```python
from build123d import *

# Parameters (mm, degrees)
BOSS_EXTRUDE1_DEPTH              = 19.05
CUT_EXTRUDE2_DEPTH               = 7658.473916494
FILLET1_R                        = 76.2
FILLET2_R                        = 31.75
SKETCH2_W                        = 127
SKETCH2_H                        = 19.05
CUT_EXTRUDE1_DEPTH               = 7658.473916494
F_1_4_0_25_DIAMETER_HOLE1_D      = 6.35
F_15_64_0_23438_DIAMETER_HOLE1_D = 5.953252
F_1_4_CLEARANCE_HOLE1_D          = 7.14248
HOLE1_D                          = 3.175
HOLE1_DEPTH                      = 50.8
HOLE1_CSINK_D                    = 10.16
HOLE1_CSINK_ANGLE                = 82
HOLE1_TIP                        = 0.953866233
HOLE2_D                          = 3.175
HOLE2_DEPTH                      = 38.1
HOLE2_CSINK_D                    = 10.16
HOLE2_CSINK_ANGLE                = 82
HOLE2_TIP                        = 0.953866233
HOLE3_D                          = 3.175
HOLE3_DEPTH                      = 50.8
HOLE3_CSINK_D                    = 10.16
HOLE3_CSINK_ANGLE                = 82
HOLE3_TIP                        = 0.953866233
HOLE4_D                          = 3.175
HOLE4_DEPTH                      = 38.1
HOLE4_CSINK_D                    = 10.16
HOLE4_CSINK_ANGLE                = 82
HOLE4_TIP                        = 0.953866233


with BuildPart() as part:
    # Sketch1 → Boss-Extrude1 (new body)
    with BuildSketch(Plane.XY):
        Polygon((3140.71, 6983.72999014), (2683.51, 6983.72999014), (2683.51, 6641.741886848), (3140.71, 6826.4626773), align=None)
    extrude(amount=BOSS_EXTRUDE1_DEPTH)

    # Sketch6 → Cut-Extrude2 (cut, through all)
    with BuildSketch(Plane(origin=(0, 0, 0), x_dir=(-1, 0, 0), z_dir=(0, 0, -1))):
        Polygon((-2923.76447292, 6932.92999014), (-3089.91, 6932.92999014), (-3089.91, 6860.727709955), (-2972.15765047, 6813.152672592), align=None)
        Polygon((-2925.056710658, 6794.122657646), (-2734.31, 6717.055984048), (-2734.31, 6932.92999014), (-2868.974907992, 6932.92999014), align=None)
    extrude(amount=-CUT_EXTRUDE2_DEPTH, mode=Mode.SUBTRACT)

    # Fillet1
    fillet1_edges = [part.edges().sort_by_distance(p)[0] for p in [
        (2925.056710658, 6794.122657646, 9.525),
        (2868.974907992, 6932.92999014, 9.525),
        (2734.31, 6932.92999014, 9.525),
        (2734.31, 6717.055984048, 9.525),
    ]]
    fillet(fillet1_edges, radius=FILLET1_R)

    # Fillet2
    fillet2_edges = [part.edges().sort_by_distance(p)[0] for p in [
        (2972.15765047, 6813.152672592, 9.525),
        (3089.91, 6860.727709955, 9.525),
        (3089.91, 6932.92999014, 9.525),
        (2923.76447292, 6932.92999014, 9.525),
    ]]
    fillet(fillet2_edges, radius=FILLET2_R)

    # Sketch2 → Cut-Extrude1 (cut, through all)
    with BuildSketch(Plane(origin=(0, 0, 0), x_dir=(-1, 0, 0), z_dir=(0, 0, -1))):
        with Locations((-2747.01, 6974.20499014)):
            Rectangle(SKETCH2_W, SKETCH2_H)
        with Locations((-3001.01, 6974.20499014)):
            Rectangle(SKETCH2_W, SKETCH2_H)
        Polygon((-2977.551881268, 6760.542518374), (-3095.304230798, 6808.117555738), (-3088.167975193, 6825.780408168), (-2970.415625663, 6778.205370804), align=None)
    extrude(amount=-CUT_EXTRUDE1_DEPTH, mode=Mode.SUBTRACT)

    # 1/4 (0.25) Diameter Hole1 (through all)
    with Locations(Plane(origin=(0, 0, 0), x_dir=(-1, 0, 0), z_dir=(0, 0, -1))):
        with Locations((-3088.167975193, 6825.780408168), (-2970.415625663, 6778.205370804), (-2937.51, 6964.67999014), (-3064.51, 6964.67999014), (-2810.51, 6964.67999014)):
            Hole(F_1_4_0_25_DIAMETER_HOLE1_D / 2)

    # 15/64 (0.23438) Diameter Hole1 (through all)
    with Locations(Plane.YX):
        with Locations((6692.541891629, 2721.610000001), (6945.629994921, 2721.610000001), (6945.629994921, 3115.310000001), (6851.60701674, 3115.310000001)):
            Hole(F_15_64_0_23438_DIAMETER_HOLE1_D / 2)

    # 1/4 Clearance Hole1 (through all)
    with Locations(Plane(origin=(0, 0, 0), x_dir=(-1, 0, 0), z_dir=(0, 0, -1))):
        with Locations((-2900.218040257, 6923.40499014)):
            Hole(F_1_4_CLEARANCE_HOLE1_D / 2)

    # Hole1
    with Locations(Plane(origin=(0, 7002.77999014, 247.523), x_dir=(0, 0, 1), z_dir=(0, 1, 0))):
        with Locations((0, 2696.21), (-237.998, 3089.91), (-237.998, 3039.11), (-237.998, 2962.91), (-237.998, 2912.11), (-237.998, 2835.91), (-237.998, 2785.11), (-237.998, 2708.91), (237.998, 2708.91), (237.998, 2785.11), (237.998, 2835.91), (237.998, 2912.11), (237.998, 2962.91), (237.998, 3039.11), (237.998, 3089.91), (0, 3051.81), (0, 2950.21), (0, 2797.81)):
            CounterSinkHole(HOLE1_D / 2, HOLE1_CSINK_D / 2, depth=HOLE1_DEPTH, counter_sink_angle=HOLE1_CSINK_ANGLE)
            with Locations((0, 0, -(HOLE1_DEPTH + HOLE1_TIP / 2))):  # 118° drill point
                Cone(0, HOLE1_D / 2, HOLE1_TIP, mode=Mode.SUBTRACT)

    # Hole2
    with Locations(Plane(origin=(3159.76, -4.781e-06, 247.523), x_dir=(0, 0, -1), z_dir=(1, 0, 0))):
        with Locations((-118.999, 6993.254994921), (237.998, 6993.254994921), (237.998, 6958.329994921), (237.998, 6845.512682081), (-237.998, 6993.254994921), (-237.998, 6958.329994921), (-237.998, 6845.512682081), (118.999, 6993.254994921)):
            CounterSinkHole(HOLE2_D / 2, HOLE2_CSINK_D / 2, depth=HOLE2_DEPTH, counter_sink_angle=HOLE2_CSINK_ANGLE)
            with Locations((0, 0, -(HOLE2_DEPTH + HOLE2_TIP / 2))):  # 118° drill point
                Cone(0, HOLE2_D / 2, HOLE2_TIP, mode=Mode.SUBTRACT)

    # Hole3
    with Locations(Plane(origin=(-1923.157317923, 4759.981389861, 247.523), x_dir=(0, 0, -1), z_dir=(0.37460659341595665, -0.9271838545667693, 0))):
        with Locations((237.998, 5442.50683469), (-237.998, 5442.50683469), (-237.998, 5394.88183469), (-237.998, 5318.68183469), (0, 5407.58183469), (0, 5305.98183469), (-237.998, 5267.88183469), (-237.998, 5130.866292514), (-237.998, 4993.850750338), (237.998, 4993.850750338), (237.998, 5130.866292514), (237.998, 5267.88183469), (237.998, 5318.68183469), (237.998, 5394.88183469)):
            CounterSinkHole(HOLE3_D / 2, HOLE3_CSINK_D / 2, depth=HOLE3_DEPTH, counter_sink_angle=HOLE3_CSINK_ANGLE)
            with Locations((0, 0, -(HOLE3_DEPTH + HOLE3_TIP / 2))):  # 118° drill point
                Cone(0, HOLE3_D / 2, HOLE3_TIP, mode=Mode.SUBTRACT)

    # Hole4
    with Locations(Plane(origin=(2664.46, -4.781e-06, 247.523), x_dir=(0, 0, 1), z_dir=(-1, 0, 0))):
        with Locations((-237.998, 6686.191891629), (237.998, 6686.191891629), (257.048, 6993.254994921), (218.948, 6993.254994921), (19.05, 6993.254994921), (237.998, 6939.279994921), (237.998, 6812.735943275), (-237.998, 6812.735943275), (-237.998, 6939.279994921), (-19.05, 6993.254994921), (-218.948, 6993.254994921), (-257.048, 6993.254994921)):
            CounterSinkHole(HOLE4_D / 2, HOLE4_CSINK_D / 2, depth=HOLE4_DEPTH, counter_sink_angle=HOLE4_CSINK_ANGLE)
            with Locations((0, 0, -(HOLE4_DEPTH + HOLE4_TIP / 2))):  # 118° drill point
                Cone(0, HOLE4_D / 2, HOLE4_TIP, mode=Mode.SUBTRACT)


solid = part.part
```
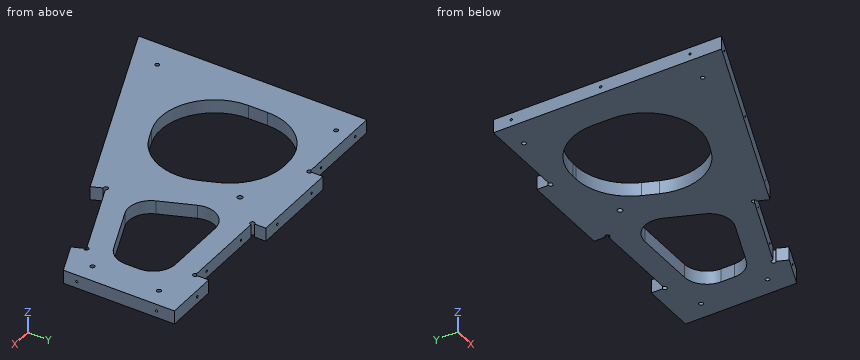
Read the model definition and answer for the solid it produces. Units are mm, in the model's axes. Round coordinates to 2 decimals unless told otherwise and drop trailing zeros. Write each loop counter-clockwise with the first axis right and the second up, starting at its lowest first coordinate (ties: lowest second). Pieces come first, ordered by that corner, then holes. Notation, with made-up numbers: (-22.5, -23) - (15.5, -23) arc R31 ccw to (15.5, 4) - close; hole circle Ø6 at (-33.75, -38.75). An arc over 180 degrees is marked (long way). One line per item, written item: value.
Q1. Each of these flat-tipped pins is pushed along its axis until it touches: P1, Ø5, axis at y = 6845.51, z = 9.53, coming from the +X side; P2, Ø8, axis at x = 3001.5, z = 16, coming from the -Y side; P3, Ø10, axis at x = 2944.5, z = 15, coming from the -Y side; P4, Ø2, axis at x = 2813.5, z = 8, coming from the -Y side. Where does it stop, or does it pass through?
The answers:
P1: stops at x = 3140.71
P2: stops at y = 6789.15
P3: stops at y = 6745.17
P4: stops at y = 6693.86
Q2. Find section A-A (x = 3075). Determine the outline of the cut face in (y, z).
The answers:
outline: (6820.46, 0) - (6855.23, 0) - (6855.23, 19.05) - (6820.46, 19.05) - close; (6928.1, 0) - (6983.73, 0) - (6983.73, 19.05) - (6928.1, 19.05) - close
Q3. Find section C-C (x = 2729.5). Determine the outline of the cut face in (y, z).
The answers:
outline: (6660.32, 0) - (6964.68, 0) - (6964.68, 19.05) - (6660.32, 19.05) - close
Q4. Find section B-B (x = 2796.5). Determine the outline of the cut face in (y, z).
The answers:
outline: (6687.39, 0) - (6755.13, 0) - (6755.13, 19.05) - (6687.39, 19.05) - close; (6931.63, 0) - (6964.68, 0) - (6964.68, 19.05) - (6931.63, 19.05) - close
Q5. Straight lines are drawn through the part: line 1 (Z direction, x = 2962.91, y = 6955.75); line 2 (X direction, y = 6813.5, z = 13.25); line 3 (Y direction, x = 3114, z = 1). For each, find the intervals that lie inside material, in ascending order. Write a range as from..to.
The answers:
line 1: z = 0..7.94, 11.11..19.05
line 2: x = 2683.51..2736.12, 2898.59..3057.77, 3093.13..3108.63
line 3: y = 6815.67..6848.93, 6854.28..6942.96, 6948.3..6983.73
